Print and shaded views of the part. All mm, measured from the part's lowest x, y and z. A direction names the side the tool comes from. Give positions to 0.01 mm unless a question says otherwise; leave off trailing zeros. Write each loop counter-clockwise with the first axis right and the second up, starting at its lowest first coordinate (ties: lowest second). Pieces come first, ordered by that corner, then holes. Notation, with made-up numbers: (-11.75, 38) -> (25.25, 38) arc R31 cw to (25.25, 67) -> close; hole circle Ø4 at (78.25, 36.5). An arc over 180 degrees is marked (long way). Put each result on its own line as item: value.
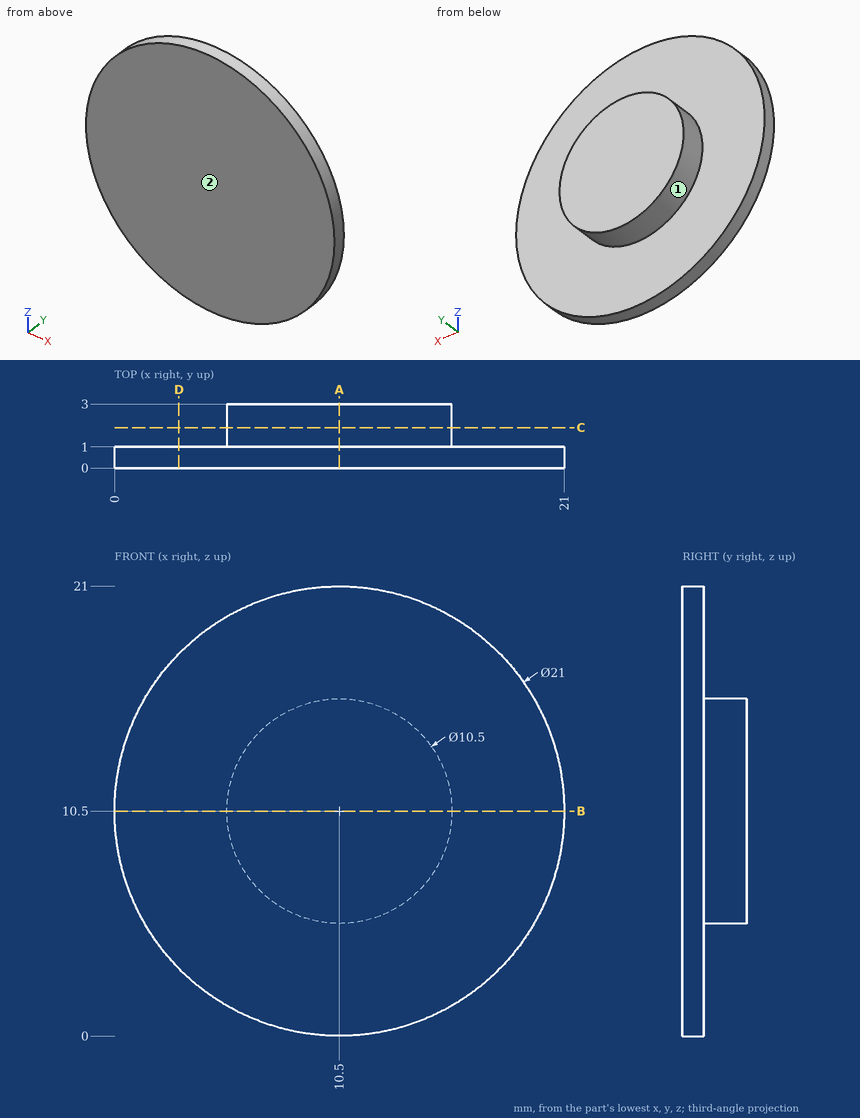
1) Slice it at A-A (x = 10.5). Write the cut outline in (y, z), plus the area to 3 significant figures.
Filled sheet:
outline: (0, 0) -> (1, 0) -> (1, 5.25) -> (3, 5.25) -> (3, 15.75) -> (1, 15.75) -> (1, 21) -> (0, 21) -> close
area: 42.0 mm2
2) Slice it at B-B (z = 10.5). Write the cut outline in (x, y), plus the area to 3 significant figures.
Filled sheet:
outline: (0, 0) -> (21, 0) -> (21, 1) -> (15.75, 1) -> (15.75, 3) -> (5.25, 3) -> (5.25, 1) -> (0, 1) -> close
area: 42.0 mm2
3) Slice it at D-D (x = 3). Write the cut outline in (y, z).
Filled sheet:
outline: (0, 3.15) -> (1, 3.15) -> (1, 17.85) -> (0, 17.85) -> close
4) Tool access for the marked faces 1 and 2: list every direction of +Z, -Z, +X, -X, +Y, -Y with a clear straight run to the whole face (end or side of a thin tool).
Filled sheet:
face 1: +Y
face 2: +Z, -Z, +X, -X, -Y
5) Pin check, flat tips, straight feed: pin 1 (1 mm diameter, centred on x = 12.5, y = 2, fed in from -Z); pin 2 (1.5 mm diameter, centred on y = 0.5, z = 16, fed in from +X); pin 3 (5 mm diameter, centred on x = 5, z = 4, fed in from +Y). Stop position of each tip, or through.
Filled sheet:
pin 1: z = 5.47
pin 2: x = 19.86
pin 3: y = 1
6) Wall check: L1, parallel to Y at x = 16.5, z = 3.75; L2, parallel to X at y = 0.4, z = 10.75; L3, parallel to X at y = 2.4, z = 8.5. Give the ranges that are in metal, low to high.
Filled sheet:
L1: 0 to 1
L2: 0 to 21
L3: 5.65 to 15.35
7) Slice it at C-C (y = 1.9). Write the cut outline in (x, z), plus the area to 3 significant figures.
Filled sheet:
outline: circle Ø10.5 at (10.5, 10.5)
area: 86.6 mm2
